Input: part model. Units: mm. Frame: model coordinates. Face numbers are marked on the shaded views. Round coordinates to 2 decimals unless told otherwise and drop trailing zeros. Loops run counter-clockwise (first coordinate to the right, second up) from the corner with the lowest first, then second, coordinate; pieces in that order, holes last. Notation, with made-up numbers: M 38.25,-33.5 L 87.25,-33.5 A22 cw 87.25,-17.5 Z; hole C 41,62 d4. An arc over 180 degrees is marked long. Return JSON: item names as keys, results as strings. Group by question number.
1) Contact query for a flat-ended pin moving along its axis: P1, Ø2, axis at x = 1, z = 13.5, coming from the +Y side. Output: stop coordinate, or through.
2) Section C-C (z = 14.25). Output: boundary loops of the cut face in (x, y).
3) Section A-A (y = 0.8). Output: boundary loops of the cut face in (x, z), plus the area to 3 significant figures.
4) Material intervals for line 1 (Z direction, x = 1.15, y = 0.4); line 2 (Y direction, x = -0.5, z = 13.5), sorted ascending. Write a range as from..to.
5) Section B-B (x = 0.5). Output: boundary loops of the cut face in (y, z).
6) Mould query, pull axis Z, two halves, no side actions, for the marked faces 1, 2, 3 and 4. Classes: +Z half, -Z half, draft (parallel to the pull), parting line (faces both ways), or undercut.
from build123d import *

# Parameters (mm, degrees)
SKETCH_1_W          = 4
SKETCH_1_H          = 4
EXTRUDE_1_DEPTH     = 30
SKETCH_4_W          = 8
SKETCH_4_H          = 2
CUT_EXTRUDE_1_DEPTH = 4


with BuildPart() as part:
    # 草圖1 → 填料-伸長1 (new body)
    with BuildSketch(Plane.XY):
        Rectangle(SKETCH_1_W, SKETCH_1_H)
    extrude(amount=EXTRUDE_1_DEPTH)

    # 草圖4 → 除料-伸長1 (cut)
    with BuildSketch(Plane.ZY.offset(2)):
        with Locations((13, 1)):
            Rectangle(SKETCH_4_W, SKETCH_4_H)
    extrude(amount=-CUT_EXTRUDE_1_DEPTH, mode=Mode.SUBTRACT)


solid = part.part
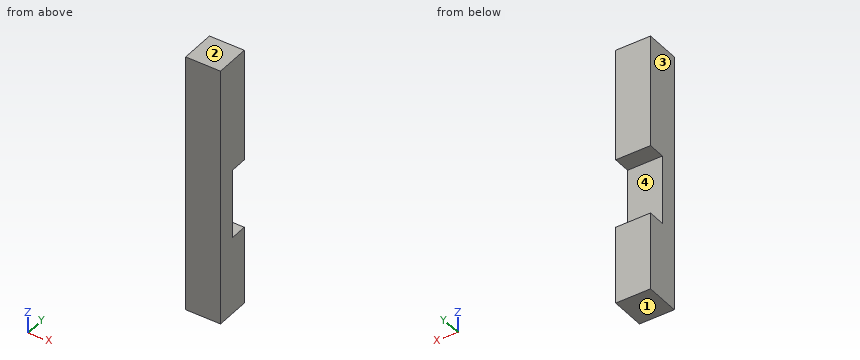
Returned:
{
 "1": {"P1": "stops at y = 0"},
 "2": {"outline": "M -2,-2 L 2,-2 L 2,0 L -2,0 Z"},
 "3": {"outline": "M -2,0 L 2,0 L 2,9 L -2,9 Z; M -2,17 L 2,17 L 2,30 L -2,30 Z", "area": "88.0 mm^2"},
 "4": {"line 1": "z = 0..9, 17..30", "line 2": "y = -2..0"},
 "5": {"outline": "M -2,0 L 2,0 L 2,9 L 0,9 L 0,17 L 2,17 L 2,30 L -2,30 Z"},
 "6": {"face 1": "-Z half", "face 2": "+Z half", "face 3": "draft", "face 4": "undercut"}
}
